Read the model definition and answer for the solid it produces. Units are mm, in the model's axes. A direction names the side the tool comes from. Give positions to 0.01 mm unless a question says otherwise; leave off trailing zeros. Loops run counter-clockwise (first coordinate to the right, second up) from the corner with the lowest first, then second, coordinate; pieces in that order, holes last. Notation, with made-up numbers: (30.25, 22.25) - (84.25, 22.25) arc R21 ccw to (84.25, 50.25) - close; hole circle Ø7 at (14.5, 66). An arc over 180 degrees is marked (long way). Put each result on its own line as item: value. Start each with the question number.
1. Given pin 1 Ø0.5 at (x, y) = (-9.5, -19) entering from -Z; pin 2 Ø2.5 at (x, y) = (0, 0) entering from +Z, each flat-ended and moving along its own axis, determine where each tip first touches the part or whether it passes through.
2. A cutting plane is placed at C-C, the plane x = 0. Determine the outline of the cut face in (y, z), plus the area to 3 significant figures.
3. A cutting plane is placed at A-A, the plane y = -14. Determine the outline of the cut face in (x, z).
4. A cutting plane is placed at B-B, the plane z = 5.4. Determine the outline of the cut face in (x, y), plus the area to 3 significant figures.
5. For faces 4 (the flat face through (0, 14.5, 5)), 5 (the flat face through (0, 13.5, 3)), 6 (the flat face through (0, -21.5, 3)), determine the directions among +Z, -Z, +X, -X, +Y, -Y from which every point of the face is accessible in a straight line to the end or side of a thin tool.
6. For a pull along X with two mould halves and no side action, classify faces 1 (the flat face through (0, -20, 6)), 2 (the cylindrical face through (-1.5, 0.07, 2.96)), 3 (the flat face through (-20, 0, 3)) as released by +X, released by -X, zero draft, split by the parting line, or undercut.
7. Consider L1, parallel to Y at x = 0, z = 2.15; L2, parallel to Y at x = -7, z = 3.5; L3, parallel to Y at x = -2.5, z = 5.1. Determine where each line is inside the solid, lowest interval first. Write a range as from..to.
8. A cutting plane is placed at D-D, the plane x = -16. Determine the outline of the cut face in (y, z).
```python
from build123d import *

# Parameters (mm, degrees)
SKETCH_1_W          = 40
SKETCH_1_H          = 43
SKETCH_1_R          = 1.5
EXTRUDE_1_DEPTH     = 6
CUT_EXTRUDE_1_DEPTH = 46.806658905


with BuildPart() as part:
    # 草图1 → 凸台-拉伸1 (new body)
    with BuildSketch(Plane.XY):
        Rectangle(SKETCH_1_W, SKETCH_1_H)
        Circle(SKETCH_1_R, mode=Mode.SUBTRACT)
    extrude(amount=EXTRUDE_1_DEPTH)

    # 草图2 → 切除-拉伸1 (cut, through all)
    with BuildSketch(Plane(origin=(20, 0, 0), x_dir=(0, 0, -1), z_dir=(1, 0, 0))):
        Polygon((-6, 18.5), (-4, 18.5), (-4, 19.5), (-2, 19.5), (-2, 13.5), (-3.925973419, 13.5), (-3.925973419, 14.5), (-6, 14.5), align=None)
        Polygon((-6, -18.5), (-6, -14.5), (-3.925973419, -14.5), (-3.925973419, -13.5), (-2, -13.5), (-2, -19.5), (-4, -19.5), (-4, -18.5), align=None)
    extrude(amount=-CUT_EXTRUDE_1_DEPTH, mode=Mode.SUBTRACT)


solid = part.part
```
Return value:
1. pin 1: stops at z = 0
1. pin 2: passes through
2. outline: (-21.5, 0) - (-1.5, 0) - (-1.5, 6) - (-14.5, 6) - (-14.5, 3.93) - (-13.5, 3.93) - (-13.5, 2) - (-19.5, 2) - (-19.5, 4) - (-18.5, 4) - (-18.5, 6) - (-21.5, 6) - close; (1.5, 0) - (21.5, 0) - (21.5, 6) - (18.5, 6) - (18.5, 4) - (19.5, 4) - (19.5, 2) - (13.5, 2) - (13.5, 3.93) - (14.5, 3.93) - (14.5, 6) - (1.5, 6) - close
2. area: 200 mm2
3. outline: (-20, 0) - (20, 0) - (20, 2) - (-20, 2) - close; (-20, 3.93) - (20, 3.93) - (20, 6) - (-20, 6) - close
4. outline: (-20, -21.5) - (20, -21.5) - (20, -18.5) - (-20, -18.5) - close; (-20, -14.5) - (20, -14.5) - (20, 14.5) - (-20, 14.5) - close; (-20, 18.5) - (20, 18.5) - (20, 21.5) - (-20, 21.5) - close; hole circle Ø3 at (0, 0)
4. area: 1,390 mm2
5. face 4: +Z, +X, -X
5. face 5: +X, -X
5. face 6: +Z, -Z, +X, -X, -Y
6. face 1: zero draft
6. face 2: undercut
6. face 3: released by -X
7. L1: y = -21.5..-19.5, -13.5..-1.5, 1.5..13.5, 19.5..21.5
7. L2: y = -21.5..-19.5, -13.5..13.5, 19.5..21.5
7. L3: y = -21.5..-18.5, -14.5..14.5, 18.5..21.5
8. outline: (-21.5, 0) - (21.5, 0) - (21.5, 6) - (18.5, 6) - (18.5, 4) - (19.5, 4) - (19.5, 2) - (13.5, 2) - (13.5, 3.93) - (14.5, 3.93) - (14.5, 6) - (-14.5, 6) - (-14.5, 3.93) - (-13.5, 3.93) - (-13.5, 2) - (-19.5, 2) - (-19.5, 4) - (-18.5, 4) - (-18.5, 6) - (-21.5, 6) - close
